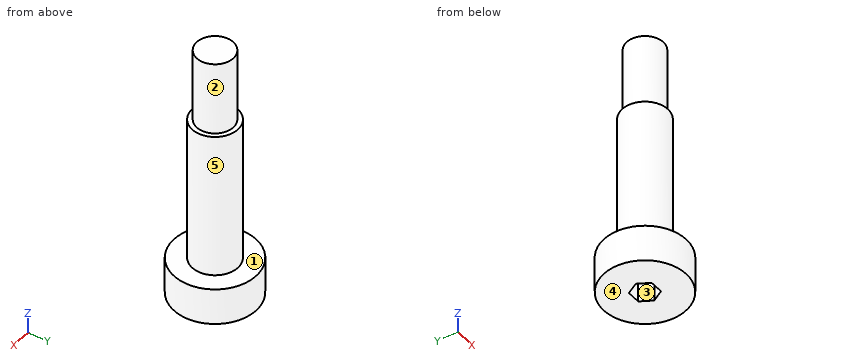
```python
from build123d import *

# Parameters (mm, degrees)
S01_GROUND_BEARING_SHOULDER_R      = 2.5
F_01_GROUND_BEARING_SHOULDER_DEPTH = 16
F_02_START                         = 16
S02_M4_RETAINING_THREAD_R          = 2
F_02_M4_RETAINING_THREAD_DEPTH     = 8
F_03_START                         = -4
S03_SOCKET_HEAD_R                  = 4.5
F_03_SOCKET_HEAD_DEPTH             = 4
F_04_START                         = -4.1
F_04_2_5_MM_HEX_KEY_DEPTH          = 2.8


with BuildPart() as part:
    # S01 - Ground bearing shoulder → 01 - Ground bearing shoulder (new body)
    with BuildSketch(Plane.XY):
        Circle(S01_GROUND_BEARING_SHOULDER_R)
    extrude(amount=F_01_GROUND_BEARING_SHOULDER_DEPTH)

    # S02 - M4 retaining thread → 02 - M4 retaining thread (add)
    with BuildSketch(Plane.XY.offset(F_02_START)):
        Circle(S02_M4_RETAINING_THREAD_R)
    extrude(amount=F_02_M4_RETAINING_THREAD_DEPTH)

    # S03 - Socket head → 03 - Socket head (add)
    with BuildSketch(Plane.XY.offset(F_03_START)):
        Circle(S03_SOCKET_HEAD_R)
    extrude(amount=F_03_SOCKET_HEAD_DEPTH)

    # S04 - 2.5 mm hex key → 04 - 2.5 mm hex key (cut)
    with BuildSketch(Plane.XY.offset(F_04_START)):
        Polygon((1.443375673, 0), (0.721687836, 1.25), (-0.721687836, 1.25), (-1.443375673, 0), (-0.721687836, -1.25), (0.721687836, -1.25), align=None)
    extrude(amount=F_04_2_5_MM_HEX_KEY_DEPTH, mode=Mode.SUBTRACT)


solid = part.part
```
Source: CAD feature listing. Evaluate the final solid. Frame: model axes, mm. Face numbers are marked on the shaded views. A direction names the side the tool comes from. Give positions to 0.01 mm unless a question says otherwise; leave off trailing zeros. Order: outer loops, then holes, each group sorted by start corner. A loop starts at its lowest first (then second) coordinate and runs counter-clockwise, first axis right, second up.
(1) Section query A-A (x = 0). Return the cut outline in (y, z).
(2) Pull-direction query (Y, two-part tool) for the marked faces 1, 2 and 3; classes: +Y half, -Y half, draft (parallel to the pull), parting line (faces both ways), or undercut.
(3) Contact query for flat-ended pins moving along their axis: P1, Ø0.7, axis at x = -0.5, z = -3, coming from the -Y side; P2, Ø4, axis at y = -3, z = 8.5, coming from the -X side; P3, Ø1, axis at x = -2.5, z = 14, coming from the +Y side. Output: stop coordinate, or through.
(4) Access query for the marked faces 4 and 5. Directions: +Z, -Z, +X, -X, +Y, -Y. A direction counts if a zero-diameter tool reaches every point of the face in a straight line with its end or side. Return the directions, or none.
(5) Section query C-C (z = 5). Return the cut outline in (x, y), plus the area to 3 significant figures.
(6) Material intervals for line 1 along Z through (x, y) = (0.25, -2.75); line 2 along Z through (x, y) = (0.25, 1); line 3 along Y through (x, z) = (-1.75, -1), sorted ascending.
(7) Section query B-B (y = 1.75). Return the cut outline in (x, z).
(8) Section query D-D (y = -1). Return the cut outline in (x, z), plus the area to 3 significant figures.
Outcome:
1. outline: (-4.5, -4) - (-1.25, -4) - (-1.25, -1.3) - (1.25, -1.3) - (1.25, -4) - (4.5, -4) - (4.5, 0) - (2.5, 0) - (2.5, 16) - (2, 16) - (2, 24) - (-2, 24) - (-2, 16) - (-2.5, 16) - (-2.5, 0) - (-4.5, 0) - close
2. face 1: draft
2. face 2: parting line
2. face 3: undercut
3. P1: stops at y = -4.5
3. P2: stops at x = -2.29
3. P3: stops at y = 1.5
4. face 4: -Z, +X, -X, +Y, -Y
4. face 5: +Z
5. outline: circle Ø5 at (0, 0)
5. area: 19.6 mm2
6. line 1: z = -4 to 0
6. line 2: z = -1.3 to 24
6. line 3: y = -4.15 to 4.15
7. outline: (-4.15, -4) - (4.15, -4) - (4.15, 0) - (1.79, 0) - (1.79, 16) - (0.97, 16) - (0.97, 24) - (-0.97, 24) - (-0.97, 16) - (-1.79, 16) - (-1.79, 0) - (-4.15, 0) - close
8. outline: (-4.39, -4) - (-0.87, -4) - (-0.87, -1.3) - (0.87, -1.3) - (0.87, -4) - (4.39, -4) - (4.39, 0) - (2.29, 0) - (2.29, 16) - (1.73, 16) - (1.73, 24) - (-1.73, 24) - (-1.73, 16) - (-2.29, 16) - (-2.29, 0) - (-4.39, 0) - close
8. area: 131 mm2
